Here's the drawing with two shaded views (mm, measured from the low corner). I have some questions. A direction names the side the tool comes from. Give positions to 0.01 mm unless a question says otherwise; leave off trailing zeros. Write each loop counter-clockwise with the first axis right and the second up, starting at its lowest first coordinate (ties: lowest second). Pieces come first, ordered by that corner, then holes. Notation, with made-up numbers: (30, 69.25) - (71, 69.25) arc R25 cw to (71, 103.25) - close; hole circle Ø9 at (3, 13.5). An arc over 180 degrees is marked (long way). Write item = value, one per line.
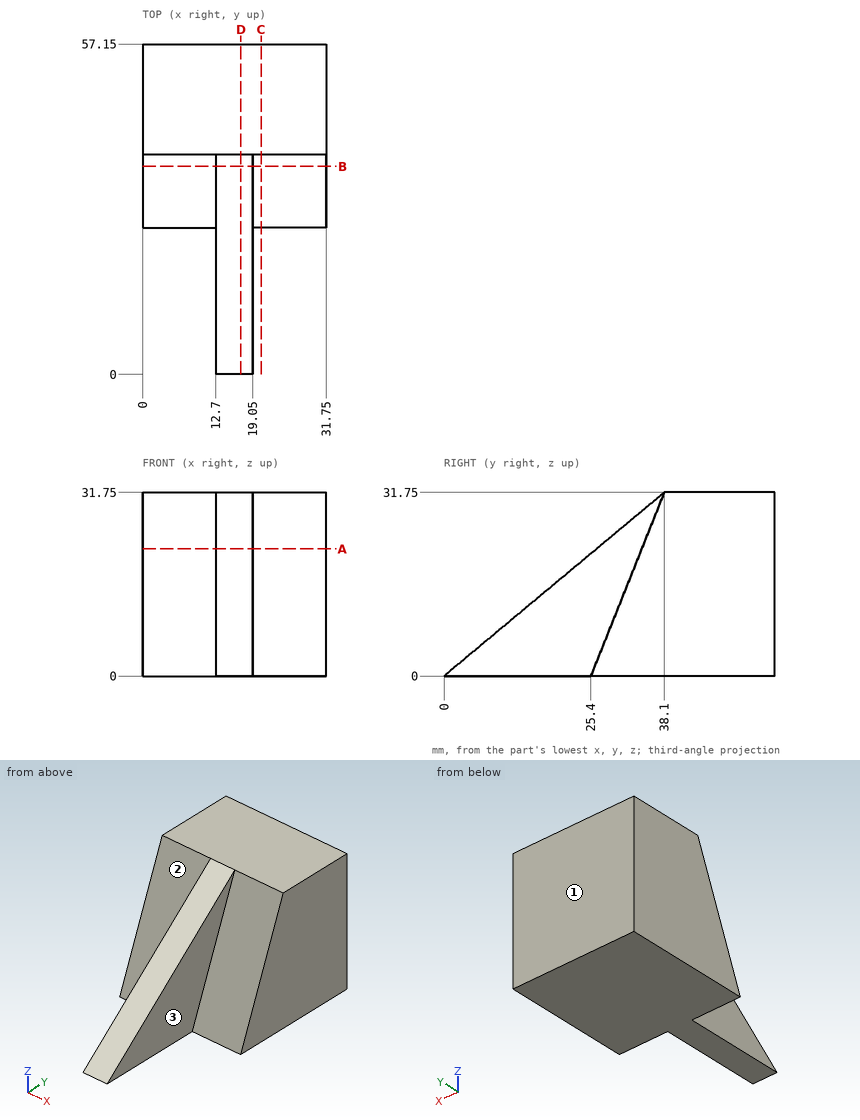
1. If we section it at C-C, the plane x = 20.5: Please give me the cut outline in (y, z).
Filled sheet:
outline = (25.4, 0) - (57.15, 0) - (57.15, 31.75) - (38.1, 31.75) - close
2. If we section it at A-A, the plane z = 22: Please give me the cut outline in (x, y), and give its area (3 significant figures).
Filled sheet:
outline = (0, 34.2) - (12.7, 34.2) - (12.7, 26.4) - (19.05, 26.4) - (19.05, 34.2) - (31.75, 34.2) - (31.75, 57.15) - (0, 57.15) - close
area = 778 mm2
3. I need wall thicknesses on line 1 (X direction, y = 19.5, z = 15.5); line 2 (Y direction, x = 11, z = 7.5); line 3 (Y direction, x = 21.5, z = 27). Which ranges of each line are inside material? Lowest first, please.
Filled sheet:
line_1 = 12.7 to 19.05
line_2 = 28.4 to 57.15
line_3 = 36.2 to 57.15
4. Which directions (+Z, -Z, +X, -X, +Y, -Y) give clear straight access to the entire face, cutting with the end or side of a thin tool? Please do the marked faces 1, 2 and 3.
Filled sheet:
face_1 = +Z, -Z, +X, -X, +Y
face_2 = +Z, -X, -Y
face_3 = +Z, +X, -Y
5. If we section it at B-B, the plane y = 36: Please give me the cut outline in (x, z).
Filled sheet:
outline = (0, 0) - (31.75, 0) - (31.75, 26.5) - (19.05, 26.5) - (19.05, 30) - (12.7, 30) - (12.7, 26.5) - (0, 26.5) - close
6. If we section it at D-D, the plane x = 17: Please give me the cut outline in (y, z).
Filled sheet:
outline = (0, 0) - (57.15, 0) - (57.15, 31.75) - (38.1, 31.75) - close
